from build123d import *

# Parameters (mm, degrees)
F0_R     = 14.2875
F0_R_2   = 6.096
F0_R_3   = 2.54
F1_DEPTH = 4.064
F2_DEPTH = 14.224
F3_R     = 2.05802


with BuildPart() as f1:
    # F0 (on Top) → F1 (new body)
    with BuildSketch(Plane.XY):
        Circle(F0_R)
        Circle(F0_R_2, mode=Mode.SUBTRACT)
        Circle(F0_R_2)
        Circle(F0_R_3, mode=Mode.SUBTRACT)
    extrude(amount=F1_DEPTH)

    # F0 (on Top) → F2 (join)
    with BuildSketch(Plane.XY):
        Circle(F0_R_2)
        Circle(F0_R_3, mode=Mode.SUBTRACT)
    extrude(amount=F2_DEPTH)

    # F3
    f3_edges = [f1.edges().sort_by_distance(p)[0] for p in [
        (-14.2875, 0, 0),
    ]]
    fillet(f3_edges, radius=F3_R)


solid = f1.part
Verification items for the finished model (mm, model axes). A direction names the side the tool comes from. Give positions to 0.01 mm unless a question says otherwise; leave off trailing zeros. Write each loop counter-clockwise with the first axis right and the second up, starting at its lowest first coordinate (ties: lowest second). Pieces come first, ordered by that corner, then holes. Notation, with made-up numbers: M 28,84.5 L 46,84.5 A22 ccw 46,116.5 Z; hole C -22.75,36.5 d3. An arc over 180 degrees is marked long. Write item = value, one per line.
(1) Sectioned sample at A-A (y = 0). Record the cut outline in (x, z), then the cut area to 3 significant figures.
Found:
outline = M -14.29,2.06 A2.06 ccw -12.23,0 L -2.54,0 L -2.54,14.22 L -6.1,14.22 L -6.1,4.06 L -14.29,4.06 Z; M 2.54,0 L 12.23,0 A2.06 ccw 14.29,2.06 L 14.29,4.06 L 6.1,4.06 L 6.1,14.22 L 2.54,14.22 Z
area = 166 mm2
(2) Material ranges on line 1 (Y direction, x = 0, z = 6.5); line 2 (X direction, y = 2.25, z = 12); line 3 (Z direction, x = -7.5, y = 7.25), recorded low to high.
Found:
line_1 = -6.1 to -2.54, 2.54 to 6.1
line_2 = -5.67 to -1.18, 1.18 to 5.67
line_3 = 0 to 4.06
(3) Draft check along Y on faces 3 (the face through (-0.794, 6.044, 9.073)), 4 (the face through (0, -3, 14.224)), 5 (the face through (-0.33, 2.52, 7.01)). Enter one of: released by +Y, released by -Y, zero draft, split by the parting line, or undercut.
Found:
face_3 = split by the parting line
face_4 = zero draft
face_5 = undercut
(4) Access from +Z, -Z, +X, -X, +Y, -Y to the whole of each face (thin tool, end or side, straight path). Record for faces 1 (the face through (-14.274, 0.628, 3.047)), 2 (the face through (6, -3, 4.064)).
Found:
face_1 = +Z, -Z
face_2 = +Z
(5) Go/stop test with flat-tipped pins: pin 1 Ø2 at (y, z) = (9.5, 1.5) entering from +X; pin 2 Ø5 at (y, z) = (2, 11) entering from -X; pin 3 Ø1.5 at (y, z) = (-2, 2.5) entering from +X; pin 4 Ø12 at (x, y) = (4, 11) entering from +Z. Record where each tip stops, or that it passes through.
Found:
pin_1 = 11.43
pin_2 = -6.1
pin_3 = 14.23
pin_4 = 14.22
(6) Sectioned sample at C-C (z = 8.5). Record the cut outline in (x, y).
Found:
outline = C 0,0 d12.19; hole C 0,0 d5.08
(7) Sectioned sample at D-D (z = 1). Record the cut outline in (x, y).
Found:
outline = C 0,0 d27.99; hole C 0,0 d5.08
